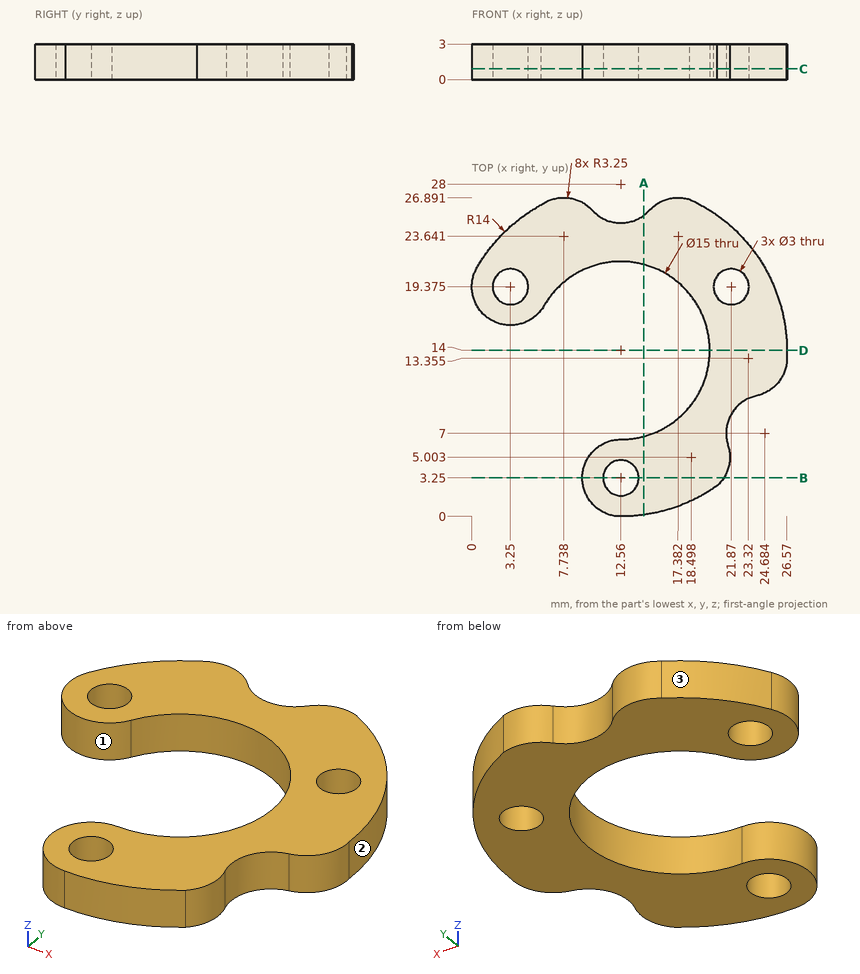
Study the drawing (mm; zero at the part's minimum x, y, z) and answer. Coordinates: 2 decimals unless noted, no trailing zeros. Write each loop counter-clockwise with the first axis right and the second up, starting at its lowest first coordinate (ties: lowest second). Pieces come first, ordered by that corner, then holes.
Q1. Section B-B, the plane y = 3.25 is taken. Write down the section's boundary in (x, z) (1 decimal).
Returned:
outline: (9.3, 0) - (11.1, 0) - (11.1, 3) - (9.3, 3) - close; (14.1, 0) - (21.2, 0) - (21.2, 3) - (14.1, 3) - close
Q2. Given P1, Ø1, axis at x = 14.5, z = 0.5, coming from the +Y side; P2, Ø1.5, axis at y = 8, z = 2.5, coming from the -X side; P3, Ø1.5, axis at x = 3, z = 1.5, coming from the +Y side, each flat-ended and moving along its own axis, determine where each tip first touches the part or whether it passes through.
Returned:
P1: stops at y = 25.85
P2: stops at x = 15.83
P3: stops at y = 24.88
Q3. Section D-D, the plane y = 14 is taken. Write down the section's boundary in (x, z).
Returned:
outline: (20.06, 0) - (26.56, 0) - (26.56, 3) - (20.06, 3) - close
Q4. Section C-C, the plane z = 0.9 is taken. Give the number of separate pieces and of enclosed holes in the cut face, then the cut area to 3 significant figures.
Returned:
separate pieces: 1
enclosed holes: 3
area: 268 mm2
Q5. Section A-A, the plane x = 14.5 is taken. Write down the section's boundary in (y, z) (1 decimal), then the cut area to 3 significant figures.
Returned:
outline: (0.1, 0) - (6.8, 0) - (6.8, 3) - (0.1, 3) - close; (21.2, 0) - (25.4, 0) - (25.4, 3) - (21.2, 3) - close
area: 32.3 mm2
Q6. Find the intervals of material crossed by line 1 along Y through (x, z) = (11.5, 2.7) (1 decimal); line 2 along Y through (x, z) = (13.5, 0.3); line 3 along X through (y, z) = (17, 2.8) (1 decimal), in increasing order.
Returned:
line 1: y = 0.2 to 2.2, 4.3 to 6.3, 21.4 to 24.9
line 2: y = 0.03 to 2.08, 4.42 to 6.56, 21.44 to 24.89
line 3: x = 1 to 5.5, 19.4 to 26.2
Q7. The mould has two halves that part along X. Classify the marked faces 1, 2 and 3: released by +X, released by -X, zero draft, split by the parting line, or undercut.
Returned:
face 1: undercut
face 2: released by +X
face 3: released by -X
